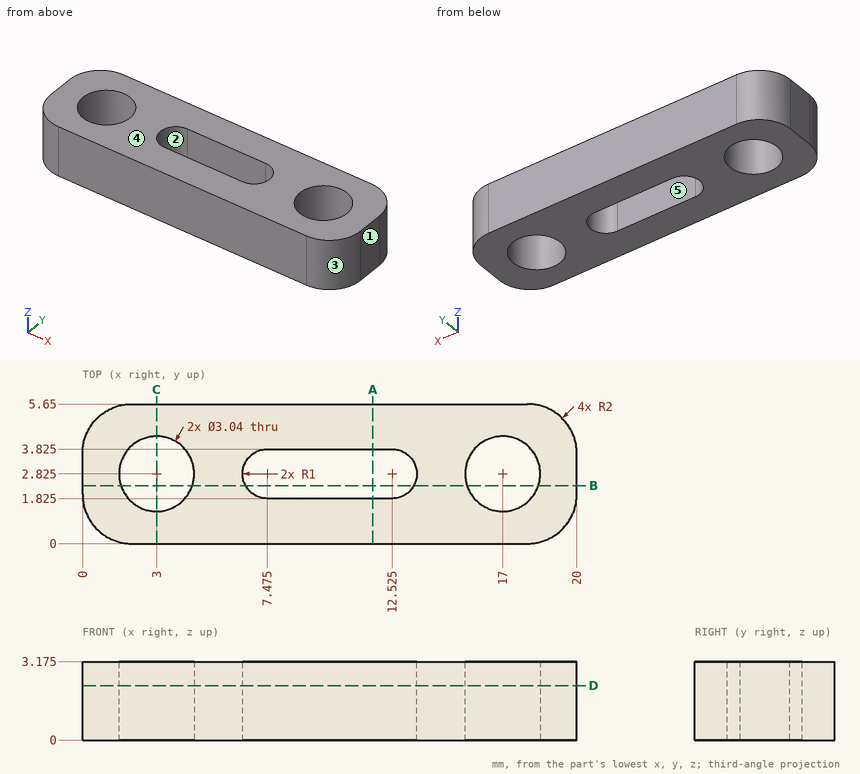
Answer from the drawing. Dimensions are ordinates in mm from the lowest x, y and z of the part. A direction names the side the tool comes from. Give positions to 0.01 mm unless a question says otherwise; leave off trailing zeros. Write each loop counter-clockwise with the first axis right and the second up, starting at its lowest first coordinate (ties: lowest second). Pieces come first, ordered by that corner, then holes. Notation, with made-up numbers: (31, 77.25) -> (72, 77.25) arc R21 cw to (72, 97.25) -> close; hole circle Ø2 at (56, 19.25). An arc over 180 degrees is marked (long way). Use a Markdown table: item, result.
(1) Section B-B, the plane y = 2.35 is taken. Determine the outline of the cut face in (x, z) (3 decimals), then the cut area to 3 significant figures.
Return value:
| item | result |
|---|---|
| outline | (0, 0) -> (1.556, 0) -> (1.556, 3.175) -> (0, 3.175) -> close; (4.444, 0) -> (6.595, 0) -> (6.595, 3.175) -> (4.444, 3.175) -> close; (13.405, 0) -> (15.556, 0) -> (15.556, 3.175) -> (13.405, 3.175) -> close; (18.444, 0) -> (20, 0) -> (20, 3.175) -> (18.444, 3.175) -> close |
| area | 23.5 mm2 |
(2) Section D-D, the plane z = 2.2 is taken. Determine the outline of the cut face in (x, y) (3 decimals).
Return value:
| item | result |
|---|---|
| outline | (0, 2) arc R2 ccw to (2, 0) -> (18, 0) arc R2 ccw to (20, 2) -> (20, 3.65) arc R2 ccw to (18, 5.65) -> (2, 5.65) arc R2 ccw to (0, 3.65) -> close; hole circle Ø3.04 at (3, 2.825); hole (7.475, 1.825) -> (12.525, 1.825) arc R1 ccw to (12.525, 3.825) -> (7.475, 3.825) arc R1 ccw to start; hole circle Ø3.04 at (17, 2.825) |
(3) Section C-C, the plane x = 3 is taken. Determine the outline of the cut face in (y, z) (3 decimals).
Return value:
| item | result |
|---|---|
| outline | (0, 0) -> (1.305, 0) -> (1.305, 3.175) -> (0, 3.175) -> close; (4.345, 0) -> (5.65, 0) -> (5.65, 3.175) -> (4.345, 3.175) -> close |
(4) A flat-ended cylindrical pin translates along its axis: P1, Ø1.8, axis at x = 17, y = 2.825, coming from the +Z side. Find the tip coordinate at first contact, or state that the pin passes through.
Return value:
| item | result |
|---|---|
| P1 | through |
(5) Find the intervals of material crossed by probe 1 along Y at (x, z) = (3, 1) (3 decimals); probe 2 along X at (y, z) = (2.35, 2.8); probe 3 along X at (y, z) = (3, 2.25), in increasing order. Write a range as from..to.
Return value:
| item | result |
|---|---|
| probe 1 | 0..1.305, 4.345..5.65 |
| probe 2 | 0..1.56, 4.44..6.6, 13.4..15.56, 18.44..20 |
| probe 3 | 0..1.49, 4.51..6.49, 13.51..15.49, 18.51..20 |
(6) Determine the mould class of the marked faces 1, 2 and 3 for opening direction Y: released by +Y, released by -Y, zero draft, split by the parting line, or undercut.
Return value:
| item | result |
|---|---|
| face 1 | zero draft |
| face 2 | undercut |
| face 3 | released by -Y |
(7) Section A-A, the plane x = 11.75 is taken. Determine the outline of the cut face in (y, z) (3 decimals), then the cut area to 3 significant figures.
Return value:
| item | result |
|---|---|
| outline | (0, 0) -> (1.825, 0) -> (1.825, 3.175) -> (0, 3.175) -> close; (3.825, 0) -> (5.65, 0) -> (5.65, 3.175) -> (3.825, 3.175) -> close |
| area | 11.6 mm2 |
(8) For the marked faces 4 and 5, determine the directions among +Z, -Z, +X, -X, +Y, -Y from which every point of the face is accessible in a straight line to the end or side of a thin tool.
Return value:
| item | result |
|---|---|
| face 4 | +Z, +X, -X, +Y, -Y |
| face 5 | +Z, -Z |
